Work out the finished part from the listing and answer in its coordinate system (mm). Coordinates: 2 decimals unless noted, no trailing zeros. Loops run counter-clockwise (first coordinate to the right, second up) from the corner with the lowest first, then second, coordinate; pieces in that order, holes last. Notation, with made-up numbers: (17, 53.5) -> (28, 53.5) arc R20 ccw to (28, 82.5) -> close; hole circle Ø3 at (69, 5.25). An arc over 180 degrees is marked (long way). Use a Markdown table: item, result. Add a question column.
Autodesk Fusion 360 part; units mm, degrees
sketch "Sketch1" plane through (0, 0, 0) normal (0, 0, 1) x (1, 0, 0)
  line L0 (0, 0) -> (-371, 0)
  line L1 (-371, 0) -> (-371, 152)
  line L2 (-371, 152) -> (0, 152)
  line L3 (0, 152) -> (0, 0)
  circle A0 centre (-366, 147) radius 1.7
  circle A1 centre (-5, 5) radius 1.7
  circle A2 centre (-366, 5) radius 1.7
  circle A3 centre (-5, 147) radius 1.7
  circle A4 centre (-366, 147) radius 3
  circle A5 centre (-5, 5) radius 3
  circle A6 centre (-366, 5) radius 3
  circle A7 centre (-5, 147) radius 3
  dimension "d1" = 371
  dimension "d2" = 152
  dimension "d3" = 3.4
  dimension "d4" = 5
  dimension "d5" = 5
  dimension "d6" = 3.4
  dimension "d7" = 3.4
  dimension "d8" = 3.4
  dimension "d9" = 5
  dimension "d10" = 5
  dimension "d11" = 5
  dimension "d12" = 5
  dimension "d13" = 5
  dimension "d14" = 5
  dimension "d15" = 6
  dimension "d16" = 6
  dimension "d17" = 6
  dimension "d18" = 6
sketch "Sketch2" plane through (0, 0, 0) normal (0, 0, 1) x (1, 0, 0)
  line L0 (-361.5, 141.5) -> (-10.5, 141.5)
  line L1 (-10.5, 141.5) -> (-10.5, 9.5)
  line L2 (-10.5, 9.5) -> (-361.5, 9.5)
  line L3 (-361.5, 9.5) -> (-361.5, 141.5)
  line L4 (0, 0) -> (-371, 0)
  line L5 (-371, 0) -> (-371, 152)
  dimension "d19" = 351
  dimension "d20" = 132
  dimension "d21" = 9.5
  dimension "d22" = 9.5
extrude "Extrude1" add sketch "Sketch1" along normal blind 5 contours L0 L1 L2 L3
extrude "Extrude2" cut sketch "Sketch2" along normal blind 10
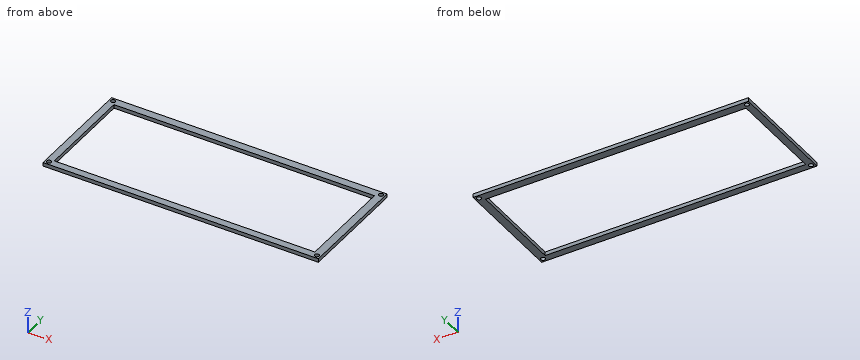
Item 1: Section C-C (y = 82.5) is taken. Determine the outline of the cut face in (x, z).
Item 2: Section B-B (z = 4.2) is taken. Determine the outline of the cut face in (x, y), then the cut area to 3 significant figures.
Item 3: Find the intervals of material crossed by probe 1 along Y at (x, z) = (-366, 3.4); probe 2 along X at (y, z) = (147, 1.3); probe 3 along Y at (x, z) = (-115, 3.95), in increasing order.
Item 4: Section A-A (x = -49) is taken. Determine the outline of the cut face in (y, z).
Output:
| question | item | result |
|---|---|---|
| 1 | outline | (-371, 0) -> (-361.5, 0) -> (-361.5, 5) -> (-371, 5) -> close; (-10.5, 0) -> (0, 0) -> (0, 5) -> (-10.5, 5) -> close |
| 2 | outline | (-371, 0) -> (0, 0) -> (0, 152) -> (-371, 152) -> close; hole circle Ø6 at (-366, 5); hole circle Ø6 at (-366, 147); hole (-361.5, 9.5) -> (-10.5, 9.5) -> (-10.5, 141.5) -> (-361.5, 141.5) -> close; hole circle Ø6 at (-5, 5); hole circle Ø6 at (-5, 147) |
| 2 | area | 9,950 mm2 |
| 3 | probe 1 | y = 0 to 2, 8 to 144, 150 to 152 |
| 3 | probe 2 | x = -371 to -369, -363 to -8, -2 to 0 |
| 3 | probe 3 | y = 0 to 9.5, 141.5 to 152 |
| 4 | outline | (0, 0) -> (9.5, 0) -> (9.5, 5) -> (0, 5) -> close; (141.5, 0) -> (152, 0) -> (152, 5) -> (141.5, 5) -> close |
